Autodesk Inventor part; units mm, degrees
ref_plane "YZ Plane" through (0, 0, 0) normal (1, 0, 0) x (0, 1, 0)
ref_plane "XZ Plane" through (0, 0, 0) normal (0, 1, 0) x (-1, 0, 0)
ref_plane "XY Plane" through (0, 0, 0) normal (0, 0, 1) x (1, 0, 0)
sketch "Sketch1" plane through (0, 0, 0) normal (0, 1, 0) x (-1, 0, 0)
  circle A0 centre (0, 0) radius 15
  dimension "d0" = 30
extrude "Extrusion1" add sketch "Sketch1" along normal blind 3
sketch "Sketch2" plane through (0, 3, 0) normal (0, 1, 0) x (1, 0, 0)
  circle A0 centre (0, 0) radius 15
  circle A1 centre (0, 0) radius 10
  dimension "d3" = 30
  dimension "d4" = 20
extrude "Extrusion2" add sketch "Sketch2" along normal blind 9
sketch "Sketch3" plane through (0, 12, 0) normal (0, 1, 0) x (1, 0, 0)
  line L0 (2.5, -15) -> (-2.5, -15)
  line L1 (-2.5, -15) -> (-2.5, 15)
  line L2 (-2.5, 15) -> (2.5, 15)
  line L3 (2.5, 15) -> (2.5, -15)
  line L4 (2.5, -15) -> (-2.5, 15) construction
  line L5 (-2.5, -15) -> (2.5, 15) construction
  point P0 (0, 0)
  dimension "d7" = 5
  dimension "d8" = 30
extrude "Extrusion3" cut sketch "Sketch3" against normal blind 8
fillet "Fillet1" radius 0.5 4 edges at (-2.5, 12, 12.2363) (-2.5, 12, -12.2363) (2.5, 12, 12.2363) (2.5, 12, -12.2363)
sketch "Sketch4" plane through (0, 3, 0) normal (0, 1, 0) x (1, 0, 0)
  circle A0 centre (0, 7) radius 1.05
  point P0 (0, 0)
  dimension "d12" = 2.1
  dimension "d13" = 7
extrude "Extrusion4" cut sketch "Sketch4" against normal through all
pattern_circular "Circular Pattern1" count 8 over 360 about axis through (0, -10, 0) along (0, 1, 0) of "Extrusion4"
sketch "Sketch5" plane through (0, 3, 0) normal (0, 1, 0) x (1, 0, 0)
  circle A0 centre (0, 0) radius 3.5
  dimension "d19" = 7
extrude "Extrusion5" cut sketch "Sketch5" against normal blind 10
properties part number "nozzle_motor_bracket"
Build history of the part. All positions in model axes, mm. A direction names the side the tool comes from. Coordinates: 2 decimals unless noted, no trailing zeros. Write each loop counter-clockwise with the first axis right and the second up, starting at its lowest first coordinate (ties: lowest second). Pieces come first, ordered by that corner, then holes.
(1) 3-axis set-ups, long thin cutter, end or side, ignore diameter. For faces 4 (the flat face through (10.2, 12, -0.2)), 5 (the flat face through (-4, 3, 0)), 6 (the flat face through (0, 4, 12)): which of +Z, -Z, +X, -X, +Y, -Y reach the whole face in a straight line?
(2) Pin check, flat tips, straight feed: pin 1 Ø8 at (x, z) = (0, 0) entering from +Y; pin 2 Ø4 at (y, z) = (9.5, 13) entering from -X; pin 3 Ø1.5 at (x, z) = (-1, -13) entering from +Y; pin 4 Ø1.7 at (x, z) = (-7, 0) entering from +Y. Stop position of each tip, or through.
(3) Cut at C-C on z = -3. List the corners of the cut face in (x, y).
(4) Cut at B-B on y = 5. List the corners of the cut face in (x, z).
(5) Drill centre lines: line 1 (Z direction, x = 0, y = 0.7); line 2 (X direction, y = 4.5, z = -3). Where is each one in solid material? Low to high.
(6) Cut at D-D on z = -7. List the corners of the cut face in (x, y), and give its area (3 significant figures).
(7) Mould opens along Z. For faces 1 (the cylindrical face through (0.989, 3.249, 14.967)), 2 (the flat face through (-10.4, 12, -0.2)), 3 (the cylindrical face through (3.95, 1.52, 4.63)) say: pulls with the +Z half, pulls with the -Z half, needs draft (parallel to the pull), parting line crosses it, or undercut.
Working result:
1. face 4: +Z, -Z, +X, -X, +Y
1. face 5: +Y
1. face 6: +Z, -Z, +Y
2. pin 1: stops at y = 3
2. pin 2: stops at x = -10.2
2. pin 3: stops at y = 4
2. pin 4: passes through
3. outline: (-14.7, 0) - (-1.8, 0) - (-1.8, 3) - (-9.54, 3) - (-9.54, 12) - (-14.7, 12) - close; (1.8, 0) - (14.7, 0) - (14.7, 12) - (9.54, 12) - (9.54, 3) - (1.8, 3) - close
4. outline: (-2.5, -14.79) - (-2.5, -9.68) arc R10 cw to (-2.5, 9.68) - (-2.5, 14.79) arc R15 ccw to start; (2.5, -14.79) arc R15 ccw to (2.5, 14.79) - (2.5, 9.68) arc R10 cw to (2.5, -9.68) - close
5. line 1: z = -15 to -8.05, -5.95 to -3.5, 3.5 to 5.95, 8.05 to 15
5. line 2: x = -14.7 to -9.54, 9.54 to 14.7
6. outline: (-13.27, 0) - (-1.05, 0) - (-1.05, 3) - (-7.14, 3) - (-7.14, 12) - (-13.27, 12) - close; (1.05, 0) - (13.27, 0) - (13.27, 12) - (7.14, 12) - (7.14, 3) - (1.05, 3) - close
6. area: 184 mm2
7. face 1: parting line crosses it
7. face 2: needs draft
7. face 3: undercut
